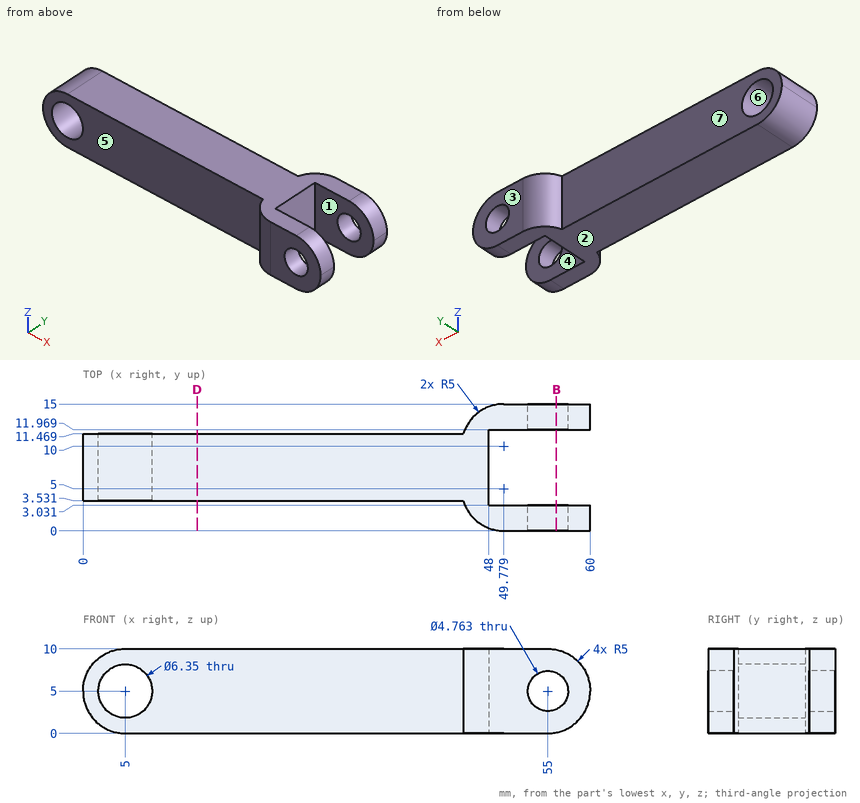
Check sheet for the drawn part. Datum: minimum x, y, z corner. Units: mm. A direction names the side the tool comes from. Round coordinates to 2 decimals unless told otherwise and drop trailing zeros. Write each loop counter-clockwise with the first axis right and the second up, starting at its lowest first coordinate (ties: lowest second). Pieces come first, ordered by that corner, then holes. Notation, with made-up numbers: (40, 13.25) - (61, 13.25) arc R14 ccw to (61, 32.25) - close; hole circle Ø1 at (-25.5, 8). An arc over 180 degrees is marked (long way). Write each question's results on one line, items separated by ' | '.
(1) Sectioned sample at B-B, the plane x = 56. Enter the section's corners in (y, z), plus the area to 3 significant figures.
Computed:
outline: (0, 0.1) - (3.03, 0.1) - (3.03, 2.84) - (0, 2.84) - close; (0, 7.16) - (3.03, 7.16) - (3.03, 9.9) - (0, 9.9) - close; (11.97, 0.1) - (15, 0.1) - (15, 2.84) - (11.97, 2.84) - close; (11.97, 7.16) - (15, 7.16) - (15, 9.9) - (11.97, 9.9) - close | area: 33.2 mm^2
(2) Set-up check for the marked faces 4, 5, 6 and 7: record each of +Z, -Z, +X, -X, +Y, -Y from which the full face is reachable in a straight line by a thin tool's end or side.
Computed:
face 4: +Z, -Z, +X | face 5: +Z, -Z, -X, -Y | face 6: +Y, -Y | face 7: +Z, -Z, -X, +Y
(3) Draft check along Y on the marked faces 1, 2 and 3. Enter one of: pulls with the +Y half, pulls with the -Y half, needs draft (parallel to the pull), parting line crosses it, or undercut.
Computed:
face 1: undercut | face 2: needs draft | face 3: pulls with the +Y half
(4) Sectioned sample at D-D, the plane x = 13.5. Enter the section's corners in (y, z).
Computed:
outline: (3.53, 0) - (11.47, 0) - (11.47, 10) - (3.53, 10) - close
(5) Thickness scan on probe 1 along X at (y, z) = (6, 5) (1 decimal); probe 2 along X at (y, z) = (1.2, 5); probe 3 along Y at (x, z) = (23.5, 1.25). Record the ranges inside material, lowest first. Write a range as from..to.
Computed:
probe 1: x = 0..1.8, 8.2..48 | probe 2: x = 46.53..52.62, 57.38..60 | probe 3: y = 3.53..11.47
(6) Depth check by flat-ended pin: pin 1 Ø5 at (x, z) = (45, 7.5) entering from -Y; pin 2 Ø4 at (x, z) = (55, 5) entering from +Y; pin 3 Ø4 at (x, z) = (20, 3.5) entering from +Y; pin 4 Ø5 at (y, z) = (4.5, 9) entering from +X. Enter the tip coordinate at first touch or a pass-through.
Computed:
pin 1: stops at y = 0.55 | pin 2: passes through | pin 3: stops at y = 11.47 | pin 4: stops at x = 59.59
